Part print with two shaded views. Sizes in mm from the minimum x, y, z corner. A direction names the side the tool comes from. Coordinates: 2 decimals unless noted, no trailing zeros. Loops run counter-clockwise (first coordinate to the right, second up) from the corner with the lowest first, then second, coordinate; pieces in that order, holes last.
(1) Slice it at A-A (y = 28). Give the cut face in (x, z).
(2) Flat gauge pins, fed straight in: P1, Ø2, axis at x = 13.5, y = 3.5, coming from the +Z side; P2, Ø0.8, axis at y = 21, z = 4.5, coming from the -X side; P3, Ø1.5, axis at y = 28.5, z = 2.5, coming from the +X side; P4, Ø1.5, axis at x = 26.5, z = 3, coming from the -Y side. Where does each tip first touch, or does it go through?
(3) Slice it at D-D (x = 23). Give the cut face in (y, z), and give its area (3 significant figures).
(4) Two-plate mould, pull along Y, no slides. Class the marked faces 5, 6, 7 and 8: pulls with the +Y half, pulls with the -Y half, needs draft (parallel to the pull), parting line crosses it, or undercut.
(5) Slice it at B-B (z = 1.1). Give the cut face in (x, y), and give its area (3 significant figures).
(6) Wall check: L1, parallel to X at y = 1.75, z = 3.85; L2, parallel to Y at x = 15, z = 3.15; L3, parallel to Y at x = 3.25, z = 1.75. Give the ranges that are in metal, low to high.
(7) Tool access for the marked faces 1, 2, 3 and 4: list every direction of +Z, -Z, +X, -X, +Y, -Y with a clear straight run to the whole face (end or side of a thin tool).
(8) Slice it at C-C (x = 15). Give the cut face in (y, z).
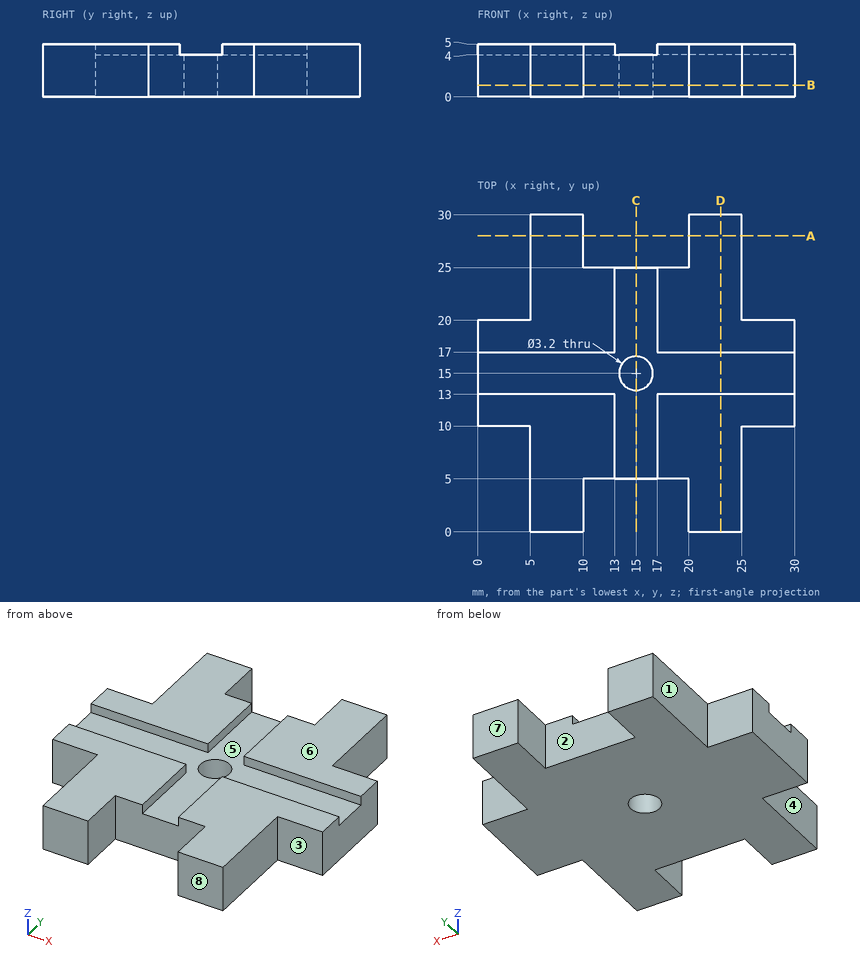
Response values:
1. outline: (5, 0) - (10, 0) - (10, 5) - (5, 5) - close; (20, 0) - (25, 0) - (25, 5) - (20, 5) - close
2. P1: passes through
2. P2: stops at x = 5
2. P3: stops at x = 25
2. P4: stops at y = 10
3. outline: (0, 0) - (30, 0) - (30, 5) - (17, 5) - (17, 4) - (13, 4) - (13, 5) - (0, 5) - close
3. area: 146 mm2
4. face 5: undercut
4. face 6: needs draft
4. face 7: pulls with the +Y half
4. face 8: pulls with the -Y half
5. outline: (0, 10) - (5, 10) - (5, 0) - (10, 0) - (10, 5) - (20, 5) - (20, 0) - (25, 0) - (25, 10) - (30, 10) - (30, 20) - (25, 20) - (25, 30) - (20, 30) - (20, 25) - (10, 25) - (10, 30) - (5, 30) - (5, 20) - (0, 20) - close; hole circle Ø3.2 at (15, 15)
5. area: 592 mm2
6. L1: x = 5 to 10, 20 to 25
6. L2: y = 5 to 13.4, 16.6 to 25
6. L3: y = 10 to 20
7. face 1: +Z, -Z, -X, +Y
7. face 2: +Z, -Z, +Y
7. face 3: +Z, -Z, +X, -Y
7. face 4: +Z, -Z, -X, -Y
8. outline: (5, 0) - (13.4, 0) - (13.4, 4) - (5, 4) - close; (16.6, 0) - (25, 0) - (25, 4) - (16.6, 4) - close
